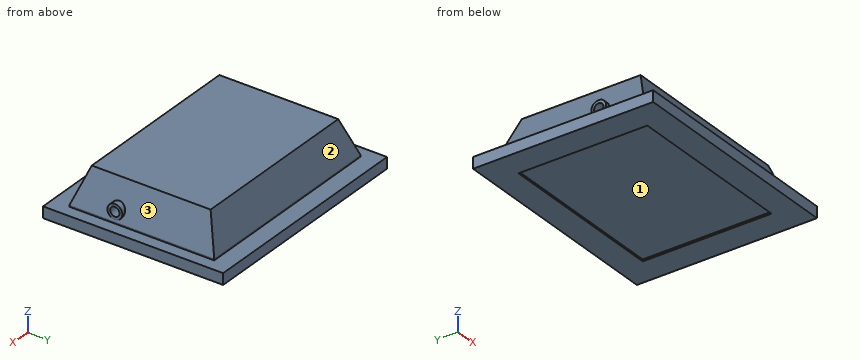
from build123d import *

# Parameters (mm, degrees)
SKIZZE1_W                       = 122
SKIZZE1_H                       = 97
AUFSATZ_LINEAR_AUSTRAGEN1_DEPTH = 6
SKIZZE2_W                       = 109
SKIZZE2_H                       = 78
AUFSATZ_LINEAR_AUSTRAGEN2_DEPTH = 20
SCHNITT_LINEAR_AUSTRAGEN1_REACH = 129.939
SKIZZE3_R                       = 2.5
FASE1_SIZE                      = 19.232341936
FASE1_SIZE_2                    = 7
AUFSATZ_LINEAR_AUSTRAGEN3_REACH = 129.939
SKIZZE4_R                       = 4
SKIZZE4_R_2                     = 2.5
SKIZZE5_W                       = 92.481860848
SKIZZE5_H                       = 69.364192104
SCHNITT_LINEAR_AUSTRAGEN2_DEPTH = 1


with BuildPart() as part:
    # Skizze1 → Aufsatz-Linear austragen1 (new body)
    with BuildSketch(Plane.XY):
        Rectangle(SKIZZE1_W, SKIZZE1_H)
    extrude(amount=AUFSATZ_LINEAR_AUSTRAGEN1_DEPTH)

    # Skizze2 → Aufsatz-Linear austragen2 (add)
    with BuildSketch(Plane.XY.offset(6)):
        Rectangle(SKIZZE2_W, SKIZZE2_H)
    extrude(amount=AUFSATZ_LINEAR_AUSTRAGEN2_DEPTH)

    # Skizze3 → Schnitt-Linear austragen1 (cut, up to next)
    with BuildSketch(Plane(origin=(54.5, 0, 0), x_dir=(0, 0, -1), z_dir=(1, 0, 0)), mode=Mode.PRIVATE) as schnitt_linear_austragen1_sk1:
        with Locations((-12, -14.5)):
            Circle(SKIZZE3_R)
    schnitt_linear_austragen1_tool1 = extrude(schnitt_linear_austragen1_sk1.sketch, amount=-SCHNITT_LINEAR_AUSTRAGEN1_REACH, mode=Mode.PRIVATE) & part.part
    add(schnitt_linear_austragen1_tool1.solids().sort_by_distance((54.5, -14.5, 12))[0], mode=Mode.SUBTRACT)

    # Fase1
    # the kernel refuses this chamfer: 19.232341936, 7 mm, written as the material it takes off along each edge
    with BuildSketch(Plane(origin=(54.5, -88.892440145, 26), x_dir=(0.013184058198645607, 0, -0.9999130865277316), z_dir=(0, 1, 0)), Plane(origin=(-54.5, 88.892440145, 26), x_dir=(-0.013184058198645607, 0, -0.9999130865277316), z_dir=(0, -1, 0))) as fase1_piece_1:
        Polygon((FASE1_SIZE * 0.999913086537, FASE1_SIZE * 0.0131840581988), (-FASE1_SIZE_2 * 0.0131840581986, FASE1_SIZE_2 * 0.999913086528), (0, 0), align=None)
    extrude(amount=177.784880291, mode=Mode.SUBTRACT)
    with BuildSketch(Plane(origin=(104.392440145, 39, 26), x_dir=(0, 0.013184058198645607, -0.9999130865277316), z_dir=(-1, 0, 0)), Plane(origin=(-104.392440145, -39, 26), x_dir=(0, -0.013184058198645607, -0.9999130865277316), z_dir=(1, 0, 0))) as fase1_piece_2:
        Polygon((FASE1_SIZE * 0.999913086537, FASE1_SIZE * 0.0131840581988), (-FASE1_SIZE_2 * 0.0131840581986, FASE1_SIZE_2 * 0.999913086528), (0, 0), align=None)
    extrude(amount=208.784880291, mode=Mode.SUBTRACT)

    # Aufsatz-Linear austragen3: up to this face of the body (flat: up to its plane)
    aufsatz_linear_austragen3_end = Plane(part.part.faces().sort_by_distance((-54.5, 0, 6.383829032))[0])
    # Skizze4 → Aufsatz-Linear austragen3 (add, up to the picked face)
    with BuildSketch(Plane(origin=(54.5, 0, 0), x_dir=(0, 0, -1), z_dir=(1, 0, 0)), mode=Mode.PRIVATE) as aufsatz_linear_austragen3_sk1:
        with Locations((-12, -14.5)):
            Circle(SKIZZE4_R)
        with Locations((-12, -14.5)):
            Circle(SKIZZE4_R_2, mode=Mode.SUBTRACT)
    aufsatz_linear_austragen3_tool1 = split(extrude(aufsatz_linear_austragen3_sk1.sketch, amount=-AUFSATZ_LINEAR_AUSTRAGEN3_REACH, mode=Mode.PRIVATE), bisect_by=aufsatz_linear_austragen3_end, keep=Keep.BOTH, mode=Mode.PRIVATE)
    add(aufsatz_linear_austragen3_tool1.solids().sort_by(Axis((54.5, -14.5, 15.886863), (-1, 0, 0)))[0])

    # Skizze5 → Schnitt-Linear austragen2 (cut)
    with BuildSketch(Plane(origin=(0, 0, 0), x_dir=(-1, 0, 0), z_dir=(0, 0, -1))):
        Rectangle(SKIZZE5_W, SKIZZE5_H)
    extrude(amount=-SCHNITT_LINEAR_AUSTRAGEN2_DEPTH, mode=Mode.SUBTRACT)


solid = part.part
Input: part model. Units: mm. Frame: model coordinates. Face numbers are marked on the shaded views. Coordinates: 2 decimals unless noted, no trailing zeros. Loops run counter-clockwise (first coordinate to the right, second up) from the corner with the lowest first, then second, coordinate; pieces in that order, holes last.
(1) Section B-B on y = -20.5. Return the cut outline in (x, z).
(2) First-contact query: pin 1 Ø2.5 at (y, z) = (-12.5, 10.5) entering from -X; pin 2 Ø2 at (y, z) = (-31.5, 18) entering from +X; pin 3 Ø6.5 at (y, z) = (-14.5, 12) entering from +X. Flat tips, straight axial feed; report the tip coordinate or a pass-through.
(3) Section A-A on x = -16. Return the cut outline in (y, z).
(4) Material intervals for probe 1 along X at (y, z) = (28, 23.25); probe 2 along Z at (x, y) = (31.5, -10); probe 3 along Y at (x, z) = (5, 12), sorted ascending.
(5) Pull-direction query (Y, two-part tool) for the marked faces 1, 2 and 3; classes: released by +Y, released by -Y, zero draft, split by the parting line, or undercut.
(6) Section C-C on z = 12. Return the cut outline in (x, y).
(7) Section D-D on y = 37. Return the cut outline in (x, z).
Data:
1. outline: (-61, 0) - (-46.24, 0) - (-46.24, 1) - (46.24, 1) - (46.24, 0) - (61, 0) - (61, 6) - (54.5, 6) - (54.5, 6.77) - (47.5, 26) - (-47.5, 26) - (-54.5, 6.77) - (-54.5, 6) - (-61, 6) - close
2. pin 1: stops at x = -54.5
2. pin 2: stops at x = 50.78
2. pin 3: stops at x = 54.5
3. outline: (-48.5, 0) - (-34.68, 0) - (-34.68, 1) - (34.68, 1) - (34.68, 0) - (48.5, 0) - (48.5, 6) - (39, 6) - (39, 6.77) - (32, 26) - (-32, 26) - (-39, 6.77) - (-39, 6) - (-48.5, 6) - close; hole circle Ø5 at (-14.5, 12)
4. probe 1: x = -48.5 to 48.5
4. probe 2: z = 1 to 26
4. probe 3: y = -37.1 to -17, -12 to 37.1
5. face 1: undercut
5. face 2: released by +Y
5. face 3: zero draft
6. outline: (-54.5, -18.5) - (-52.6, -18.5) - (-52.6, -37.1) - (52.6, -37.1) - (52.6, -18.5) - (54.5, -18.5) - (54.5, -17) - (-54.5, -17) - close; (-54.5, -12) - (54.5, -12) - (54.5, -10.5) - (52.6, -10.5) - (52.6, 37.1) - (-52.6, 37.1) - (-52.6, -10.5) - (-54.5, -10.5) - close
7. outline: (-61, 0) - (61, 0) - (61, 6) - (54.5, 6) - (54.5, 6.77) - (52.5, 12.26) - (-52.5, 12.26) - (-54.5, 6.77) - (-54.5, 6) - (-61, 6) - close
